The listing builds one solid part. Answer for the finished solid, in the listing's coordinates (mm). Give positions to 0.01 mm unless a question says otherwise; leave off trailing zeros. Order: outer loops, then holes, each group sorted by start corner. A loop starts at its lowest first (then second) coordinate and runs counter-clockwise, first axis right, second up. Notation, with made-up numbers: (20, -2.5) - (67, -2.5) arc R24 ccw to (67, 10.5) - close; hole circle Ø1 at (81.5, -15.5). An arc over 180 degrees is marked (long way). Answer as CSV lines item,"result". Start each with the question number.
1. Section B-B on z = 18.75 is taken. Give the vertices of the cut face in (x, y), and give its area (3 significant figures).
2. Section C-C on x = 12 is taken. Give the vertices of the cut face in (y, z).
3. Consider line 1 along Y through (x, z) = (35.5, 13.25); line 2 along X through (y, z) = (-19, 13.5); line 3 along Y through (x, z) = (-4, 22.25). Determine where each line is inside the solid, lowest interval first. Write a range as [from, to].
4. Section D-D on x = -53.5 is taken. Give the vertices of the cut face in (y, z), and give its area (3 significant figures).
5. Section A-A on y = 0 is taken. Give the vertices of the cut face in (x, z).
6. Flat-ended cylindrical pins translate along their axes: pin 1 (2 mm diameter, centred on y = 16.5, z = 22.5, fed in from +X); pin 2 (12 mm diameter, centred on x = 43.5, z = 19, fed in from -Y). Find the tip coordinate at first contact, or state that the pin passes through.
from build123d import *

# Parameters (mm, degrees)
F0_W     = 127
F0_H     = 76.2
F1_DEPTH = 25.4
F2_R     = 2.5
F3_DEPTH = 25.4
F4_R     = 12.7


with BuildPart() as f1:
    # F0 (on Top) → F1 (new body)
    with BuildSketch(Plane.XY):
        Rectangle(F0_W, F0_H)
    extrude(amount=F1_DEPTH)

    # F2 (on face) → F3 (cut)
    with BuildSketch(Plane.XY.offset(25.4)):
        with Locations((-2.076801, 0)):
            Circle(F2_R)
    extrude(amount=-F3_DEPTH, mode=Mode.SUBTRACT)

    # F4
    f4_edges = [f1.edges().sort_by_distance(p)[0] for p in [
        (63.5, 0, 25.4),
        (0, 38.1, 25.4),
        (0, -38.1, 25.4),
        (-63.5, 0, 25.4),
    ]]
    fillet(f4_edges, radius=F4_R)


solid = f1.part
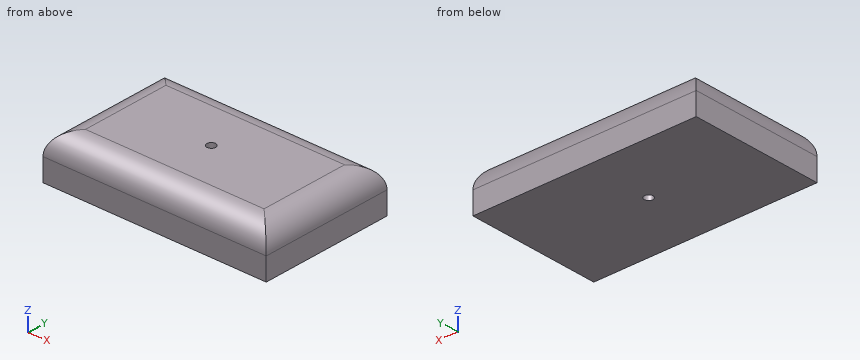
Checks:
1,outline,"(-61.97, -36.57) - (61.97, -36.57) - (61.97, 36.57) - (-61.97, 36.57) - close; hole circle Ø5 at (-2.08, 0)"
1,area,"9,040 mm²"
2,outline,"(-38.1, 0) - (38.1, 0) - (38.1, 12.7) arc R12.7 ccw to (25.4, 25.4) - (-25.4, 25.4) arc R12.7 ccw to (-38.1, 12.7) - close"
3,line 1,"y = [-38.09, 38.09]"
3,line 2,"x = [-63.47, 63.47]"
3,line 3,"y = [-33.77, -1.6], [1.6, 33.77]"
4,outline,"(-38.1, 0) - (38.1, 0) - (38.1, 12.7) arc R12.7 ccw to (28.1, 25.11) - (-28.1, 25.11) arc R12.7 ccw to (-38.1, 12.7) - close"
4,area,"1,850 mm²"
5,outline,"(-63.5, 0) - (-4.58, 0) - (-4.58, 25.4) - (-50.8, 25.4) arc R12.7 ccw to (-63.5, 12.7) - close; (0.42, 0) - (63.5, 0) - (63.5, 12.7) arc R12.7 ccw to (50.8, 25.4) - (0.42, 25.4) - close"
6,pin 1,"stops at x = 59.96"
6,pin 2,"stops at y = -38.1"
